Check sheet for the modelled part. Datum: model origin and axes. Units: mm. A direction names the side the tool comes from. Coordinates: 2 decimals unless noted, no trailing zeros. Loops run counter-clockwise (first coordinate to the right, second up) from the corner with the lowest first, then second, coordinate; pieces in that order, holes last. Notation, with made-up numbers: M 30,-36 L 38,-36 A27 ccw 38,-20 Z; hole C 57.25,67.5 d5. An arc over 180 degrees is marked long. Write each question's results on one line, items separated by ' | '. Start each with the question number.
from build123d import *

# Parameters (mm, degrees)
SKETCH1_W               = 22.5
SKETCH1_H               = 17.5
BOSS_EXTRUDE1_DEPTH     = 10
CUT_EXTRUDE1_DEPTH      = 24.082731641
CUT_EXTRUDE1_DEPTH_BACK = 24.082731641
SKETCH2_R               = 1.825
CUT_EXTRUDE2_DEPTH      = 13.5
CUT_EXTRUDE3_REACH      = 19.405
SKETCH4_W               = 11.529065942
SKETCH4_H               = 13.5
FILLET1_R               = 3


with BuildPart() as part:
    # Sketch1 → Boss-Extrude1 (new body)
    with BuildSketch(Plane(origin=(0, 0, 0), x_dir=(1, 0, 0), z_dir=(0, 1, 0))):
        Rectangle(SKETCH1_W, SKETCH1_H)
    extrude(amount=BOSS_EXTRUDE1_DEPTH)

    # Sketch2 → Cut-Extrude1 (cut, two sides: drawn at the far end of the back side and taken through both)
    with BuildSketch(Plane.XY.offset(8.75).offset(-CUT_EXTRUDE1_DEPTH_BACK)):
        with Locations((0, 6)):
            Circle(SKETCH2_R)
        with BuildLine():
            Line((-11.25, 5), (-11.25, 0))
            Line((-11.25, 0), (11.25, 0))
            Line((11.25, 0), (11.25, 5))
            ThreePointArc((11.25, 5), (0, 0.01), (-11.25, 5))
        make_face()
    extrude(amount=CUT_EXTRUDE1_DEPTH + CUT_EXTRUDE1_DEPTH_BACK, mode=Mode.SUBTRACT)

    # Sketch3 → Cut-Extrude2 (cut)
    with BuildSketch(Plane.XY.offset(6.75)):
        with BuildLine():
            ThreePointArc((-9.233945582, 9.952114837), (0, 0.969656164), (9.233945582, 9.952114837))
            ThreePointArc((9.233945582, 9.952114837), (7.547885163, 11.733945582), (5.766054418, 10.047885163))
            ThreePointArc((5.766054418, 10.047885163), (0, 4.438869486), (-5.766054418, 10.047885163))
            ThreePointArc((-5.766054418, 10.047885163), (-7.547885163, 11.733945582), (-9.233945582, 9.952114837))
        make_face()
    extrude(amount=-CUT_EXTRUDE2_DEPTH, mode=Mode.SUBTRACT)

    # Sketch4 → Cut-Extrude3 (cut, up to next)
    with BuildSketch(Plane(origin=(0, 10, 0), x_dir=(1, 0, 0), z_dir=(0, 1, 0)), mode=Mode.PRIVATE) as cut_extrude3_sk1:
        Rectangle(SKETCH4_W, SKETCH4_H)
    cut_extrude3_tool1 = extrude(cut_extrude3_sk1.sketch, amount=-CUT_EXTRUDE3_REACH, mode=Mode.PRIVATE) & part.part
    add(cut_extrude3_tool1.solids().sort_by_distance((0, 10, 0))[0], mode=Mode.SUBTRACT)

    # Fillet1
    # the kernel refuses this fillet: 3 mm, written as the material it takes off along each edge
    with BuildSketch(Plane(origin=(11.25, 5, 12.185069568), x_dir=(0, 1, 0), z_dir=(0, 0, -1))) as fillet1_piece_1:
        with BuildLine():
            CenterArc((1.230754269, -3), FILLET1_R, 90, 47.349204062)
            ThreePointArc((-0.975735859, -0.967415115), (-0.498821765, -0.472659508), (0, 0))
            Line((0, 0), (1.230754269, 0))
        make_face()
    extrude(amount=24.370139136, mode=Mode.SUBTRACT)
    with BuildSketch(Plane(origin=(-11.25, 5, 12.185069568), x_dir=(0, 1, 0), z_dir=(0, 0, -1))) as fillet1_piece_2:
        with BuildLine():
            CenterArc((1.230754269, 3), FILLET1_R, 222.650795938, 47.349204062)
            ThreePointArc((-0.975735859, 0.967415115), (-0.498821765, 0.472659508), (0, 0))
            Line((0, 0), (1.230754269, 0))
        make_face()
    extrude(amount=24.370139136, mode=Mode.SUBTRACT)
    with BuildSketch(Plane(origin=(11.25, 10, -16.25), x_dir=(-1, 0, 0), z_dir=(0, 0, 1))) as fillet1_piece_3:
        with BuildLine():
            CenterArc((FILLET1_R, FILLET1_R), FILLET1_R, 180, 90)
            Line((0, FILLET1_R), (0, 0))
            Line((0, 0), (FILLET1_R, 0))
        make_face()
    extrude(amount=32.5, mode=Mode.SUBTRACT)
    with BuildSketch(Plane(origin=(-11.25, 10, 16.25), x_dir=(0, -1, 0), z_dir=(0, 0, -1))) as fillet1_piece_4:
        with BuildLine():
            CenterArc((FILLET1_R, -FILLET1_R), FILLET1_R, 90, 90)
            Line((0, -FILLET1_R), (0, 0))
            Line((0, 0), (FILLET1_R, 0))
        make_face()
    extrude(amount=32.5, mode=Mode.SUBTRACT)


solid = part.part
Item 1: Depth check by flat-ended pin: P1, Ø1.5, axis at x = -4, z = -3, coming from the +Y side; P2, Ø6, axis at x = 5.5, z = -2.5, coming from the -Y side; P3, Ø1.5, axis at y = 4, z = 4, coming from the +X side. Enter the tip coordinate at first touch or a pass-through.
Item 2: Section check C-C (y = 5.25). Record the cut outline in (x, z).
Item 3: Thickness scan on line 1 (Z direction, x = -5.5, y = 6); line 2 (X direction, y = 5, z = 5); line 3 (X direction, y = 6.75, z = -4). Record the ranges inside material, lowest first.
Item 4: Release check for a two-part mould opening along Y. For faces 3 (the face through (1.74, 6.55, -7.76)), 4 (the face through (0, 4, 8.75)), 5 (the face through (0, 10, 8)) record: +Y half, -Y half, draft (parallel to the pull), parting line (faces both ways), or undercut.
Item 5: Section check D-D (x = -8.5). Record the cut outline in (y, z), plus the area to 3 significant figures.
Item 6: Section check A-A (x = 0). Record the cut outline in (y, z) (3 decimals), plus the area to 3 significant figures.
Item 7: Tool access check on faces 1 (the face through (-0.2, 0.97, 0.09)), 2 (the face through (-10.73, 8.69, 0.12)). Record the directions out of +Z, -Z, +X, -X, +Y, -Y that give a thin tool (end or side, any length) a straight path to the whole face; none if there is none.
Computed values:
1) P1: stops at y = 2.28 | P2: stops at y = 0.22 | P3: stops at x = 10.86
2) outline: M -11.09,-8.75 L -1.66,-8.75 L -1.66,-6.75 L -7.79,-6.75 L -7.79,6.75 L -1.66,6.75 L -1.66,8.75 L -11.09,8.75 Z; M 1.66,-8.75 L 11.09,-8.75 L 11.09,8.75 L 1.66,8.75 L 1.66,6.75 L 7.79,6.75 L 7.79,-6.75 L 1.66,-6.75 Z
3) line 1: z = -8.75 to -6.75, 6.75 to 8.75 | line 2: x = -10.99 to -7.63, 7.63 to 10.99 | line 3: x = -11.25 to -8.57, 8.57 to 11.25
4) face 3: undercut | face 4: draft | face 5: +Y half
5) outline: M 2.61,-8.75 L 9.99,-8.75 L 9.99,-6.75 L 6.59,-6.75 L 6.59,6.75 L 9.99,6.75 L 9.99,8.75 L 2.61,8.75 Z | area: 83.2 mm²
6) outline: M 0.01,-8.75 L 4.175,-8.75 L 4.175,-6.75 L 0.97,-6.75 L 0.97,6.75 L 4.175,6.75 L 4.175,8.75 L 0.01,8.75 Z; M 7.825,-8.75 L 10,-8.75 L 10,-6.75 L 7.825,-6.75 Z; M 7.825,6.75 L 10,6.75 L 10,8.75 L 7.825,8.75 Z | area: 38.3 mm²
7) face 1: +Y | face 2: +Z, -Z, -X, +Y
